Part model, mm, in its own coordinate system. A direction names the side the tool comes from. Give positions to 0.01 mm unless a question says otherwise; leave off trailing zeros. Order: outer loops, then holes, each group sorted by start corner. A loop starts at its lowest first (then second) coordinate and runs counter-clockwise, first axis right, second up. Notation, with made-up numbers: (47, 18.25) - (83, 18.25) arc R18 ccw to (83, 48.25) - close; hole circle Ø1 at (-9.75, 30.25). An arc over 180 degrees is marked (long way). Use a Markdown table: item, result. Add a question column.
Autodesk Inventor part; units mm, degrees
ref_plane "YZ Plane" through (0, 0, 0) normal (1, 0, 0) x (0, 1, 0)
ref_plane "XZ Plane" through (0, 0, 0) normal (0, 1, 0) x (-1, 0, 0)
ref_plane "XY Plane" through (0, 0, 0) normal (0, 0, 1) x (1, 0, 0)
sketch "Sketch1" plane through (0, 0, 0) normal (0, 1, 0) x (-1, 0, 0)
  line L0 (57.7037, 0.576) -> (-56.5963, 0.576)
  line L1 (-56.5963, 0.576) -> (-56.5963, 41.851)
  line L2 (-56.5963, 41.851) -> (57.7037, 41.851)
  line L3 (57.7037, 41.851) -> (57.7037, 0.576)
  point P0 (0, 0)
  dimension "d0" = 114.3
  dimension "d1" = 41.275
extrude "Extrusion1" add sketch "Sketch1" along normal blind 3.175
sketch "Sketch2" plane through (0, 3.175, 0) normal (0, 1, 0) x (1, 0, 0)
  line L0 (56.5963, -0.576) -> (-57.7037, -0.576)
  line L1 (-57.7037, -0.576) -> (56.5963, -0.576)
  line L2 (56.5963, -0.576) -> (56.5963, -3.751)
  line L3 (56.5963, -3.751) -> (-57.7037, -3.751)
  line L4 (-57.7037, -3.751) -> (-57.7037, -0.576)
  point P0 (0, 0)
  dimension "d4" = 3.175
  dimension "d5" = 114.3
extrude "Extrusion2" add sketch "Sketch2" along normal blind 101.6
sketch "Sketch3" plane through (0, 3.175, 0) normal (0, 1, 0) x (1, 0, 0)
  line L0 (-57.7037, -41.851) -> (56.5963, -41.851)
  line L1 (-57.7037, -41.851) -> (56.5963, -41.851)
  line L2 (56.5963, -41.851) -> (56.5963, -38.676)
  line L3 (56.5963, -38.676) -> (-57.7037, -38.676)
  line L4 (-57.7037, -38.676) -> (-57.7037, -41.851)
  point P0 (0, 0)
  dimension "d8" = 3.175
  dimension "d9" = 114.3
extrude "Extrusion3" add sketch "Sketch3" along normal blind 101.6
sketch "Sketch4" plane through (0, 3.175, 0) normal (0, 1, 0) x (1, 0, 0)
  line L0 (-57.7037, -3.751) -> (-57.7037, -38.676)
  line L1 (-57.7037, -3.751) -> (-54.5287, -3.751)
  line L2 (-54.5287, -3.751) -> (-54.5287, -38.676)
  line L3 (-54.5287, -38.676) -> (-57.7037, -38.676)
  line L4 (-57.7037, -38.676) -> (-57.7037, -3.751)
  point P0 (0, 0)
  dimension "d12" = 3.175
  dimension "d13" = 34.925
extrude "Extrusion4" add sketch "Sketch4" along normal blind 101.6
sketch "Sketch5" plane through (0, 3.175, 0) normal (0, 1, 0) x (1, 0, 0)
  line L0 (-54.5287, -3.751) -> (56.5963, -3.751)
  line L1 (56.5963, -3.751) -> (53.4213, -3.751)
  line L2 (53.4213, -3.751) -> (53.4213, -38.676)
  line L3 (53.4213, -38.676) -> (56.5963, -38.676)
  line L4 (56.5963, -38.676) -> (56.5963, -3.751)
  point P0 (0, 0)
  dimension "d16" = 3.175
  dimension "d17" = 34.925
extrude "Extrusion5" add sketch "Sketch5" along normal blind 101.6
sketch "Sketch6" plane through (0, 3.175, 0) normal (0, 1, 0) x (1, 0, 0)
  line L0 (-54.5287, -38.676) -> (-54.5287, -3.751)
  line L1 (-54.5287, -3.751) -> (53.4213, -3.751)
  line L2 (-54.5287, -3.751) -> (53.4213, -3.751)
  line L3 (53.4213, -3.751) -> (53.4213, -6.926)
  line L4 (53.4213, -6.926) -> (-54.5287, -6.926)
  line L5 (-54.5287, -6.926) -> (-54.5287, -3.751)
  point P0 (0, 0)
  point P1 (-54.5287, -6.926)
  dimension "d20" = 107.95
  dimension "d21" = 3.175
extrude "Extrusion6" add sketch "Sketch6" along normal blind 12.7
sketch "Sketch7" plane through (0, 3.175, 0) normal (0, 1, 0) x (1, 0, 0)
  line L0 (-54.5287, -38.676) -> (53.4213, -38.676)
  line L1 (-54.5287, -38.676) -> (53.4213, -38.676)
  line L2 (53.4213, -38.676) -> (53.4213, -35.501)
  line L3 (53.4213, -35.501) -> (-54.5287, -35.501)
  line L4 (-54.5287, -35.501) -> (-54.5287, -38.676)
  point P0 (0, 0)
  dimension "d24" = 3.175
  dimension "d25" = 107.95
extrude "Extrusion7" add sketch "Sketch7" along normal blind 12.7
sketch "Sketch9" plane through (0, 3.175, 0) normal (0, 1, 0) x (1, 0, 0)
  line L0 (-54.5287, -6.926) -> (53.4213, -6.926)
  line L1 (-54.5287, -6.926) -> (-51.3537, -6.926)
  line L2 (-51.3537, -6.926) -> (-51.3537, -35.501)
  line L3 (-51.3537, -35.501) -> (-54.5287, -35.501)
  line L4 (-54.5287, -35.501) -> (-54.5287, -6.926)
  point P0 (0, 0)
  dimension "d30" = 3.175
  dimension "d31" = 28.575
extrude "Extrusion8" add sketch "Sketch9" along normal blind 12.7
sketch "Sketch10" plane through (0, 3.175, 0) normal (0, 1, 0) x (1, 0, 0)
  line L0 (53.4213, -3.751) -> (53.4213, -6.926)
  line L1 (-54.5287, -6.926) -> (53.4213, -6.926)
  line L2 (53.4213, -6.926) -> (50.2463, -6.926)
  line L3 (50.2463, -6.926) -> (50.2463, -35.501)
  line L4 (50.2463, -35.501) -> (53.4213, -35.501)
  line L5 (53.4213, -35.501) -> (53.4213, -6.926)
  point P0 (0, 0)
  point P1 (-51.3537, -6.926)
  dimension "d34" = 3.175
  dimension "d35" = 28.575
extrude "Extrusion9" add sketch "Sketch10" along normal blind 12.7
sketch "Sketch11" plane through (0, 0, 0) normal (0, -1, 0) x (1, 0, 0)
  line L0 (56.5963, 41.851) -> (56.5963, 0.576)
  line L1 (56.5963, 41.851) -> (56.5963, 21.2135)
  line L2 (56.5963, 21.2135) -> (-0.5537, 21.2135)
  point P0 (0, 0)
  dimension "d38" = 20.6375
  dimension "d39" = 57.15
hole "Hole1" at (-0.5537, 0, 21.2135) direction (0, 1, 0) diameter 12.7 end through all
properties part number "five_cell_bottom_case"
1. Cut at D-D (x = -38). Write the cut outline in (y, z) (3 decimals), plus the area to 3 significant figures.
2. Cut at B-B (x = -3.5). Write the cut outline in (y, z) (3 decimals).
3. Cut at A-A (y = 25). Write the cut outline in (x, z), plus the area to 3 significant figures.
4. Cut at C-C (z = 10). Write the cut outline in (x, y) (3 decimals).
5. Tool access for faces 1 (the face through (-1, 52, 0.576)), 2 (the face through (0, 9, 6.926)): list every direction of +Z, -Z, +X, -X, +Y, -Y with a clear straight run to the whole face (end or side of a thin tool).
6. Drill centre lines: probe 1 along Z at (x, y) = (-32, 9); probe 2 along Z at (x, y) = (24, 75.5); probe 3 along X at (y, z) = (24.5, 10). Where is each one in solid material? Low to high. Write a range as [from, to].
7. Mould opens along Z. For faces 3 (the face through (-57.704, 52, 21)), 4 (the face through (-1, 52, 41.851)), 5 (the face through (0, 3.175, 28)) say: released by +Z, released by -Z, zero draft, split by the parting line, or undercut.
8. Pin check, flat tips, straight feed: P1, Ø10.5, axis at x = 4, z = 20, coming from the +Y side (3 decimals); P2, Ø23, axis at x = 14.5, z = 27, coming from the +Y side (3 decimals). Stop position of each tip, or through.
Responses:
| question | item | result |
|---|---|---|
| 1 | outline | (0, 0.576) - (104.775, 0.576) - (104.775, 3.751) - (15.875, 3.751) - (15.875, 6.926) - (3.175, 6.926) - (3.175, 35.501) - (15.875, 35.501) - (15.875, 38.676) - (104.775, 38.676) - (104.775, 41.851) - (0, 41.851) - close |
| 1 | area | 857 mm² |
| 2 | outline | (0, 0.576) - (104.775, 0.576) - (104.775, 3.751) - (15.875, 3.751) - (15.875, 6.926) - (3.175, 6.926) - (3.175, 15.588) - (0, 15.588) - close; (0, 26.839) - (3.175, 26.839) - (3.175, 35.501) - (15.875, 35.501) - (15.875, 38.676) - (104.775, 38.676) - (104.775, 41.851) - (0, 41.851) - close |
| 3 | outline | (-57.7, 0.58) - (56.6, 0.58) - (56.6, 41.85) - (-57.7, 41.85) - close; hole (-54.53, 3.75) - (53.42, 3.75) - (53.42, 38.68) - (-54.53, 38.68) - close |
| 3 | area | 948 mm² |
| 4 | outline | (-57.704, 0) - (56.596, 0) - (56.596, 104.775) - (53.421, 104.775) - (53.421, 15.875) - (50.246, 15.875) - (50.246, 3.175) - (-51.354, 3.175) - (-51.354, 15.875) - (-54.529, 15.875) - (-54.529, 104.775) - (-57.704, 104.775) - close |
| 5 | face 1 | -Z, +X, -X, +Y, -Y |
| 5 | face 2 | +Y |
| 6 | probe 1 | z = [0.58, 6.93], [35.5, 41.85] |
| 6 | probe 2 | z = [0.58, 3.75], [38.68, 41.85] |
| 6 | probe 3 | x = [-57.7, -54.53], [53.42, 56.6] |
| 7 | face 3 | zero draft |
| 7 | face 4 | released by +Z |
| 7 | face 5 | undercut |
| 8 | P1 | stops at y = 3.175 |
| 8 | P2 | stops at y = 15.875 |
